Autodesk Inventor part; units mm, degrees
ref_plane "YZ Plane" through (0, 0, 0) normal (1, 0, 0) x (0, 1, 0)
ref_plane "XZ Plane" through (0, 0, 0) normal (0, 1, 0) x (-1, 0, 0)
ref_plane "XY Plane" through (0, 0, 0) normal (0, 0, 1) x (1, 0, 0)
sketch "Sketch1" plane through (0, 0, 0) normal (0, 1, 0) x (-1, 0, 0)
  line L0 (8.2561, 0) -> (4.1281, -7.15)
  line L1 (4.1281, -7.15) -> (-4.1281, -7.15)
  line L2 (-4.1281, -7.15) -> (-8.2561, 0)
  line L3 (-8.2561, 0) -> (-4.1281, 7.15)
  line L4 (-4.1281, 7.15) -> (4.1281, 7.15)
  line L5 (4.1281, 7.15) -> (8.2561, 0)
  point P0 (0, 0)
  point P1 (0, 0)
  dimension "d0" = 14.3
extrude "Extrusion1" add sketch "Sketch1" along normal blind 6.35
sketch "Sketch2" plane through (0, 6.35, 0) normal (0, 1, 0) x (1, 0, 0)
  circle A0 centre (0, 0) radius 4.765
  dimension "d3" = 9.53
extrude "Extrusion2" cut sketch "Sketch2" against normal through all
thread "Thread1"
chamfer "Chamfer1" distance 0.254 angle 45 2 edges at (-4.765, 0, 0) (-4.765, 6.35, 0)
sketch "Sketch3" plane through (0, 6.35, 0) normal (0, 1, 0) x (1, 0, 0)
  circle A0 centre (0, 0) radius 7.15
  line L0 (-8.2561, 0) -> (-4.1281, -7.15)
extrude "Extrusion3" cut sketch "Sketch3" against normal blind 6.35 draft 45 keep common part
sketch "Sketch4" plane through (0, 0, 0) normal (0, -1, 0) x (1, 0, 0)
  arc A0 (0, 7.15) -> (-6.1921, 3.575) centre (0, 0) ccw
  circle A1 centre (0, 0) radius 7.15
  point P0 (0, 7.15)
extrude "Extrusion4" cut sketch "Sketch4" against normal blind 6.35 draft 45 keep common part
properties part number "Nut" material "Stainless Steel"
Model file for the job. Use its own axes, mm. Give positions to 0.01 mm unless a question says otherwise; leave off trailing zeros. Loops run counter-clockwise (first coordinate to the right, second up) from the corner with the lowest first, then second, coordinate; pieces in that order, holes last. Notation, with made-up numbers: (26.5, -8) - (81.5, -8) arc R20 ccw to (81.5, -2) - close; hole circle Ø11 at (23, 11.5). An arc over 180 degrees is marked (long way). One line per item, written item: value. Start each with the question number.
1. Slice it at B-B (y = 0.75). List the corners of the cut face in (x, z) (3 decimals).
2. Slice it at A-A (y = 3.75). List the corners of the cut face in (x, z) (3 decimals), plus the area to 3 significant figures.
3. Pull direction X, two halves, no side cores. Call faces 1 (the flat face through (2, 0, 5)), 2 (the cylindrical face through (-0.62, 3.216, -4.724)), 3 (the conical face through (-3.725, 6.081, -6.416)), 4 (the conical face through (7.4, 6.1, 0)): pulls with the +X half, pulls with the -X half, needs draft (parallel to the pull), parting line crosses it, or undercut.
4. Probe L1, parallel to Z at x = 0, y = 2.5 (3 decimals); L2, parallel to Z at x = -0.75, y = 3.5; L3, parallel to X at y = 3.75, z = 4. List the from-to ranges inside material, lowest first. Write a range as from..to.
Solution:
1. outline: (-7.872, -0.665) - (-4.512, -6.485) arc R7.9 ccw to (-3.36, -7.15) - (3.36, -7.15) arc R7.9 ccw to (4.512, -6.485) - (7.872, -0.665) arc R7.9 ccw to (7.872, 0.665) - (4.512, 6.485) arc R7.9 ccw to (3.36, 7.15) - (-3.36, 7.15) arc R7.9 ccw to (-4.512, 6.485) - (-7.872, 0.665) arc R7.9 ccw to start; hole circle Ø9.53 at (0, 0)
2. outline: (-8.256, 0) - (-4.128, -7.15) - (4.128, -7.15) - (8.256, 0) - (4.128, 7.15) - (-4.128, 7.15) - close; hole circle Ø9.53 at (0, 0)
2. area: 106 mm^2
3. face 1: needs draft
3. face 2: undercut
3. face 3: pulls with the -X half
3. face 4: pulls with the +X half
4. L1: z = -7.15..-4.765, 4.765..7.15
4. L2: z = -7.15..-4.71, 4.71..7.15
4. L3: x = -5.95..-2.59, 2.59..5.95
